from build123d import *

# Parameters (mm, degrees)
F0_W     = 38.1
F0_H     = 88.9
F1_DEPTH = 914.4
F2_R     = 3.175
F4_W     = 38.1
F4_H     = 95.25
F5_DEPTH = 76.2


with BuildPart() as f1:
    # F0 (on Right) → F1 (new body, symmetric)
    with BuildSketch(Plane.YZ):
        Rectangle(F0_W, F0_H)
    extrude(amount=F1_DEPTH, both=True)

    # F2
    f2_edges = [f1.edges().sort_by_distance(p)[0] for p in [
        (0, -19.05, 44.45),
        (0, 19.05, 44.45),
        (0, -19.05, -44.45),
        (0, 19.05, -44.45),
    ]]
    fillet(f2_edges, radius=F2_R)

    # F4 (on face) → F5 (join)
    with BuildSketch(Plane.XZ.offset(19.05)):
        with Locations((76.2, 0)):
            Rectangle(F4_W, F4_H)
    extrude(amount=F5_DEPTH)

    # F6: F1 across plane


with BuildPart() as f1_1:
    add(f1.part)
    add(f1.part.mirror(Plane.YZ))


solid = f1_1.part
The listing builds one solid part. Answer for the finished solid, in the listing's coordinates (mm). A direction names the side the tool comes from. Coordinates: 2 decimals unless noted, no trailing zeros. Order: outer loops, then holes, each group sorted by start corner. A loop starts at its lowest first (then second) coordinate and runs counter-clockwise, first axis right, second up.
Q1. Which of the six approach directions +Z, -Z, +X, -X, +Y, -Y give full straight-line access (tool end or side, diameter ignored) to faces 1 (the face through (-499, -19.05, -1)), 2 (the face through (511, -19.05, -1)), 3 (the face through (1, -19.05, -1))?
Q2. A cutting plane is placed at A-A, the plane y = -35.5. Write down the section's boundary in (x, z) (3 decimals), and give its area (3 significant figures).
Q3. A cutting plane is placed at C-C, the plane x = 591. Write down the section's boundary in (y, z) (3 decimals), and give its area (3 significant figures).
Q4. Given P1, Ø10, axis at y = -54.5, z = -2, coming from the -X side; P2, Ø23, axis at y = -57, z = -8.5, coming from the +X side; P3, Ø4, axis at x = 695.5, y = -5, coming from the +Z side, each flat-ended and moving along its own axis, determine where each tip first touches the part or whether it passes through.
Q5. A cutting plane is placed at B-B, the plane z = -23.5. Write down the section's boundary in (x, y), and give its area (3 significant figures).
Q6. Consider line 1 (X direction, y = -51, z = 38.5); line 2 (Z direction, x = 175.5, y = 10.5); line 3 (Y direction, x = 697.5, z = 8). Determine where each line is inside the solid, lowest interval first.
Answers follow:
1. face 1: +Z, -Z, -X, -Y
1. face 2: +Z, -Z, +X, -Y
1. face 3: +Z, -Z, -Y
2. outline: (-95.25, -47.625) - (-57.15, -47.625) - (-57.15, 47.625) - (-95.25, 47.625) - close; (57.15, -47.625) - (95.25, -47.625) - (95.25, 47.625) - (57.15, 47.625) - close
2. area: 7,260 mm2
3. outline: (-19.05, -41.275) arc R3.175 ccw to (-15.875, -44.45) - (15.875, -44.45) arc R3.175 ccw to (19.05, -41.275) - (19.05, 41.275) arc R3.175 ccw to (15.875, 44.45) - (-15.875, 44.45) arc R3.175 ccw to (-19.05, 41.275) - close
3. area: 3,380 mm2
4. P1: stops at x = -95.25
4. P2: stops at x = 95.25
4. P3: stops at z = 44.45
5. outline: (-914.4, -19.05) - (-95.25, -19.05) - (-95.25, -95.25) - (-57.15, -95.25) - (-57.15, -19.05) - (57.15, -19.05) - (57.15, -95.25) - (95.25, -95.25) - (95.25, -19.05) - (914.4, -19.05) - (914.4, 19.05) - (-914.4, 19.05) - close
5. area: 75,500 mm2
6. line 1: x = -95.25 to -57.15, 57.15 to 95.25
6. line 2: z = -44.45 to 44.45
6. line 3: y = -19.05 to 19.05
